from build123d import *

# Parameters (mm, degrees)
SKETCH1_W           = 205.785682804
SKETCH1_H           = 104.534748446
BOSS_EXTRUDE1_DEPTH = 70.104
SKETCH2_W           = 145.758865666
SKETCH2_H           = 50.974097726
CUT_EXTRUDE1_DEPTH  = 25.4
SKETCH3_W           = 65.29816474
SKETCH3_H           = 24.799651417
BOSS_EXTRUDE2_DEPTH = 87.63


with BuildPart() as part:
    # Sketch1 → Boss-Extrude1 (new body)
    with BuildSketch(Plane(origin=(0, 0, 0), x_dir=(1, 0, 0), z_dir=(0, 1, 0))):
        Rectangle(SKETCH1_W, SKETCH1_H)
    extrude(amount=BOSS_EXTRUDE1_DEPTH)

    # Sketch2 → Cut-Extrude1 (cut)
    with BuildSketch(Plane(origin=(0, 70.104, 0), x_dir=(1, 0, 0), z_dir=(0, 1, 0))):
        Rectangle(SKETCH2_W, SKETCH2_H)
    extrude(amount=-CUT_EXTRUDE1_DEPTH, mode=Mode.SUBTRACT)

    # Sketch3 → Boss-Extrude2 (add)
    with BuildSketch(Plane(origin=(102.892841402, 0, 0), x_dir=(0, 0, -1), z_dir=(1, 0, 0))):
        with Locations((0, 32.321763147)):
            Rectangle(SKETCH3_W, SKETCH3_H)
    extrude(amount=BOSS_EXTRUDE2_DEPTH)


solid = part.part
Geometry check sheet. Reference: the model listing, model coordinates, mm. A direction names the side the tool comes from. Coordinates: 2 decimals unless noted, no trailing zeros. Order: outer loops, then holes, each group sorted by start corner. A loop starts at its lowest first (then second) coordinate and runs counter-clockwise, first axis right, second up. Notation, with made-up numbers: (60, 61) -> (98, 61) arc R8 cw to (98, 72) -> close; hole circle Ø5 at (-25, 3.25). An arc over 180 degrees is marked (long way). Use a Markdown table: item, result. Add a question column.
1. Cross-section at A-A (y = 54.5). Enter the section's corners in (x, z), and give its area (3 significant figures).
2. Cross-section at B-B (z = -2). Enter the section's corners in (x, y).
3. Set-up check for faces 1 (the face through (146, 19.922, 0)), 2 (the face through (-1, 44.704, 0)), 3 (the face through (146, 32, 32.649)), 4 (the face through (146, 32, -32.649)): record each of +Z, -Z, +X, -X, +Y, -Y from which the full face is reachable in a straight line by a thin tool's end or side.
4. Go/stop test with flat-tipped pins: pin 1 Ø7.5 at (x, y) = (157, 26.5) entering from +Z; pin 2 Ø3 at (y, z) = (52, -9.5) entering from +X; pin 3 Ø20 at (x, y) = (132.5, 26.5) entering from -Z. Record where each tip stops, or that it passes through.
5. Cross-section at D-D (y = 28.5). Enter the section's corners in (x, z).
6. Material ranges on L1, parallel to Z at x = -21, y = 61; L2, parallel to X at y = 48, z = -0.5; L3, parallel to X at y = 11, z = 15.5, recorded low to high.
7. Mould release check, pull along Z, two halves, no side actions. Record for faces 5 (the face through (-72.879, 58, 0)), 6 (the face through (146, 44.722, 0)), 7 (the face through (-1, 35, -52.267)): pulls with the +Z half, pulls with the -Z half, needs draft (parallel to the pull), parting line crosses it, or undercut.
8. Cross-section at C-C (x = 12). Enter the section's corners in (y, z).
Filled sheet:
| question | item | result |
|---|---|---|
| 1 | outline | (-102.89, -52.27) -> (102.89, -52.27) -> (102.89, 52.27) -> (-102.89, 52.27) -> close; hole (-72.88, -25.49) -> (72.88, -25.49) -> (72.88, 25.49) -> (-72.88, 25.49) -> close |
| 1 | area | 14,100 mm2 |
| 2 | outline | (-102.89, 0) -> (102.89, 0) -> (102.89, 19.92) -> (190.52, 19.92) -> (190.52, 44.72) -> (102.89, 44.72) -> (102.89, 70.1) -> (72.88, 70.1) -> (72.88, 44.7) -> (-72.88, 44.7) -> (-72.88, 70.1) -> (-102.89, 70.1) -> close |
| 3 | face 1 | +Z, -Z, +X, -Y |
| 3 | face 2 | +Y |
| 3 | face 3 | +Z, +X, +Y, -Y |
| 3 | face 4 | -Z, +X, +Y, -Y |
| 4 | pin 1 | z = 32.65 |
| 4 | pin 2 | x = 102.89 |
| 4 | pin 3 | z = -32.65 |
| 5 | outline | (-102.89, -52.27) -> (102.89, -52.27) -> (102.89, -32.65) -> (190.52, -32.65) -> (190.52, 32.65) -> (102.89, 32.65) -> (102.89, 52.27) -> (-102.89, 52.27) -> close |
| 6 | L1 | -52.27 to -25.49, 25.49 to 52.27 |
| 6 | L2 | -102.89 to -72.88, 72.88 to 102.89 |
| 6 | L3 | -102.89 to 102.89 |
| 7 | face 5 | undercut |
| 7 | face 6 | needs draft |
| 7 | face 7 | pulls with the -Z half |
| 8 | outline | (0, -52.27) -> (70.1, -52.27) -> (70.1, -25.49) -> (44.7, -25.49) -> (44.7, 25.49) -> (70.1, 25.49) -> (70.1, 52.27) -> (0, 52.27) -> close |
